```python
from build123d import *

# Parameters (mm, degrees)
SKETCH_1_R          = 2.9
SKETCH_1_R_2        = 1.9
EXTRUDE_1_DEPTH     = 22.1
CHAMFER_1_SIZE      = 0.5
SKETCH_3_W          = 1
SKETCH_3_H          = 1.984217256
CUT_EXTRUDE_1_DEPTH = 3.5


with BuildPart() as part:
    # 草图1 → 拉伸-薄壁1 (new body)
    with BuildSketch(Plane.XY):
        Circle(SKETCH_1_R)
        Circle(SKETCH_1_R_2, mode=Mode.SUBTRACT)
    extrude(amount=-EXTRUDE_1_DEPTH)

    # 倒角1
    chamfer_1_edges = [part.edges().sort_by_distance(p)[0] for p in [
        (-2.9, 0, -22.1),
    ]]
    chamfer(chamfer_1_edges, length=CHAMFER_1_SIZE)

    # 草图3 → 切除-拉伸1 (cut)
    with BuildSketch(Plane(origin=(0, 0, -22.1), x_dir=(-1, 0, 0), z_dir=(0, 0, -1))):
        with Locations((0, -2.273251869)):
            Rectangle(SKETCH_3_W, SKETCH_3_H)
        with Locations((0, 2.273251869)):
            Rectangle(SKETCH_3_W, SKETCH_3_H)
    extrude(amount=-CUT_EXTRUDE_1_DEPTH, mode=Mode.SUBTRACT)


solid = part.part
```
CAD build for the part. Positions are in the model's coordinates, mm. A direction names the side the tool comes from. Coordinates: 2 decimals unless noted, no trailing zeros. Order: outer loops, then holes, each group sorted by start corner. A loop starts at its lowest first (then second) coordinate and runs counter-clockwise, first axis right, second up. Notation, with made-up numbers: (20.25, 13.5) -> (44.25, 13.5) arc R32 ccw to (44.25, 49.5) -> close; hole circle Ø2 at (77.25, 19). An arc over 180 degrees is marked (long way). Use one line per item in the form item = value. Start each with the question number.
1) Band-saw the part on B-B on x = 0. Give the cut face in (y, z).
2) Pull direction X, two halves, no side cores. Call faces 1 (the flat face through (-0.5, -2, -20)), 2 (the flat face through (-2.1, 0, -22.1)), 3 (the flat face through (-0.5, 2, -20)), 4 (the cylindrical face through (-0.63, -2.83, -10.65)): +X half, -X half, draft (parallel to the pull), parting line (faces both ways), or undercut.
3) Drop flat-ended pins along their axis: pin 1 (0.8 mm diameter, centred on x = 0, y = 2.5, fed in from -Z); pin 2 (1.1 mm diameter, centred on y = 2.5, z = -19.5, fed in from +X); pin 3 (1.1 mm diameter, centred on y = 2, z = -19.5, fed in from -X). Give the stop position or say it passes through.
4) Tool access for faces 5 (the cylindrical face through (1.812, 0.571, -10.895)), 6 (the flat face through (0, 2.4, -18.6)): list every direction of +Z, -Z, +X, -X, +Y, -Y with a clear straight run to the whole face (end or side of a thin tool).
5) Band-saw the part on A-A on z = -20. Give the cut face in (x, y).
6) Band-saw the part on C-C on y = 0. Give the cut face in (x, z).
7) Drill centre lines: L1, parallel to Y at x = 0, z = -10; L2, parallel to Y at x = -1.2, z = -11.5. Where is each one in solid material? Low to high. Write a range as [from, to].
8) Band-saw the part on D-D on z = -1.5. Give the cut face in (x, y).
Entries:
q1.outline = (-2.9, -18.6) -> (-1.9, -18.6) -> (-1.9, 0) -> (-2.9, 0) -> close; (1.9, -18.6) -> (2.9, -18.6) -> (2.9, 0) -> (1.9, 0) -> close
q2.face_1 = undercut
q2.face_2 = draft
q2.face_3 = undercut
q2.face_4 = parting line
q3.pin_1 = -18.6
q3.pin_2 = 2.15
q3.pin_3 = -2.51
q4.face_5 = +Z, -Z
q4.face_6 = -Z, +Y, -Y
q5.outline = (-0.5, -2.86) -> (-0.5, -1.83) arc R1.9 cw to (-0.5, 1.83) -> (-0.5, 2.86) arc R2.9 ccw to start; (0.5, -2.86) arc R2.9 ccw to (0.5, 2.86) -> (0.5, 1.83) arc R1.9 cw to (0.5, -1.83) -> close
q6.outline = (-2.9, -21.6) -> (-2.4, -22.1) -> (-1.9, -22.1) -> (-1.9, 0) -> (-2.9, 0) -> close; (1.9, -22.1) -> (2.4, -22.1) -> (2.9, -21.6) -> (2.9, 0) -> (1.9, 0) -> close
q7.L1 = [-2.9, -1.9], [1.9, 2.9]
q7.L2 = [-2.64, -1.47], [1.47, 2.64]
q8.outline = circle Ø5.8 at (0, 0); hole circle Ø3.8 at (0, 0)
